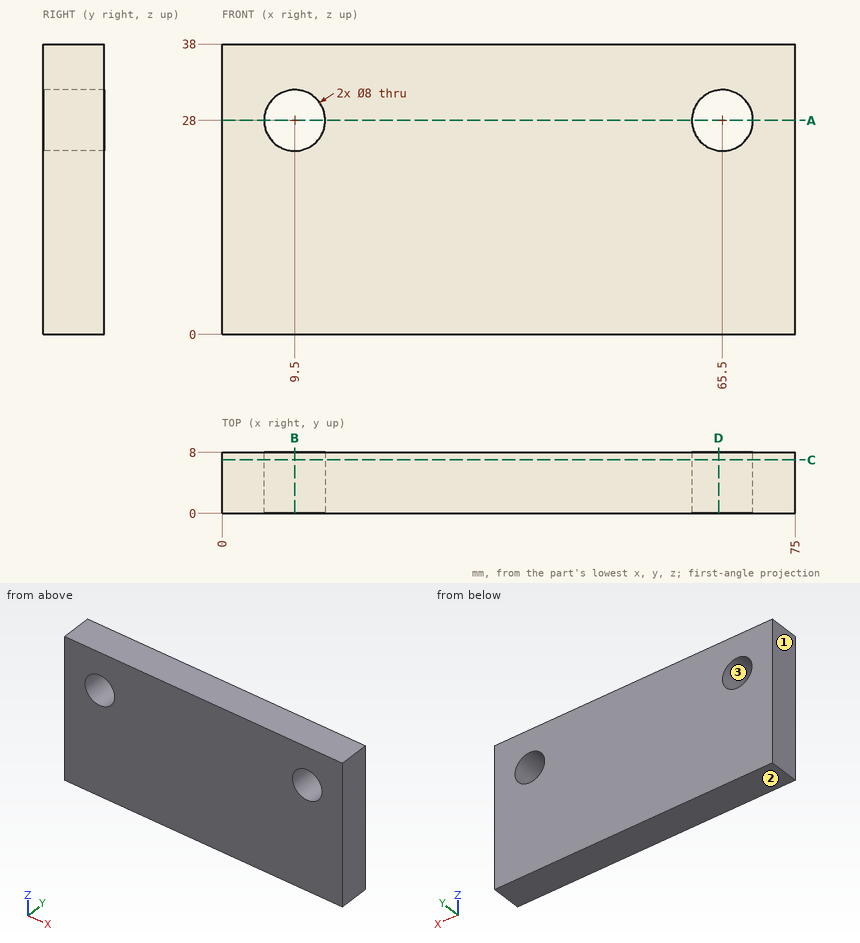
The figure shows three views and two pictorial views of one solid part (mm, origin at its lowest corner). Answer the questions. Give positions to 0.01 mm unless a question says otherwise; leave off trailing zeros. Order: outer loops, then holes, each group sorted by start corner. A loop starts at its lowest first (then second) coordinate and runs counter-clockwise, first axis right, second up. Notation, with made-up numbers: M 69.25,41.5 L 104.25,41.5 A19 cw 104.25,49.5 Z; hole C 84,2 d5. An arc over 180 degrees is marked long. Return JSON: item names as keys, results as strings.
1) Section C-C, the plane y = 7 is taken. Write down the section's boundary in (x, z), plus the area to 3 significant figures.
Resolved:
{"outline": "M 0,0 L 75,0 L 75,38 L 0,38 Z; hole C 9.5,28 d8; hole C 65.5,28 d8", "area": "2,750 mm^2"}
2) Section B-B, the plane x = 9.5 is taken. Write down the section's boundary in (y, z).
Resolved:
{"outline": "M 0,0 L 8,0 L 8,24 L 0,24 Z; M 0,32 L 8,32 L 8,38 L 0,38 Z"}
3) Straight lines are drawn through the part: line 1 along Z through (x, y) = (9.5, 2.5); line 2 along X through (y, z) = (6.75, 26); line 3 along Z through (x, y) = (13, 7.5). For each, find the intervals that lie inside material, in ascending order. Write a range as [from, to].
Resolved:
{"line 1": "[0, 24], [32, 38]", "line 2": "[0, 6.04], [12.96, 62.04], [68.96, 75]", "line 3": "[0, 26.06], [29.94, 38]"}
4) For a pull along X with two mould halves and no side action, classify the marked faces 1, 2 and 3 as +X half, -X half, draft (parallel to the pull), parting line (faces both ways), or undercut.
Resolved:
{"face 1": "-X half", "face 2": "draft", "face 3": "undercut"}
5) Section D-D, the plane x = 65 is taken. Write down the section's boundary in (y, z), plus the area to 3 significant figures.
Resolved:
{"outline": "M 0,0 L 8,0 L 8,24.03 L 0,24.03 Z; M 0,31.97 L 8,31.97 L 8,38 L 0,38 Z", "area": "241 mm^2"}
6) Section A-A, the plane z = 28 is taken. Write down the section's boundary in (x, y).
Resolved:
{"outline": "M 0,0 L 5.5,0 L 5.5,8 L 0,8 Z; M 13.5,0 L 61.5,0 L 61.5,8 L 13.5,8 Z; M 69.5,0 L 75,0 L 75,8 L 69.5,8 Z"}
